Autodesk Inventor part; units mm, degrees
ref_plane "YZ Plane" through (0, 0, 0) normal (1, 0, 0) x (0, 1, 0)
ref_plane "XZ Plane" through (0, 0, 0) normal (0, 1, 0) x (-1, 0, 0)
ref_plane "XY Plane" through (0, 0, 0) normal (0, 0, 1) x (1, 0, 0)
sketch "Sketch1" plane through (0, 0, 0) normal (0, 1, 0) x (-1, 0, 0)
  point P0 (0, 0)
sketch "Sketch2" plane through (0, 0, 0) normal (0, 1, 0) x (-1, 0, 0)
  point P0 (0, 0)
sketch "Sketch3" plane through (0, 0, 0) normal (0, 1, 0) x (-1, 0, 0)
  point P0 (0, 0)
sketch "Sketch4" plane through (0, 0, 0) normal (0, 1, 0) x (-1, 0, 0)
  line L0 (35, 20) -> (-35, 20)
  line L1 (-35, 20) -> (-35, -20)
  line L2 (-35, -20) -> (35, -20)
  line L3 (35, -20) -> (35, 20)
  line L4 (35, 20) -> (-35, -20) construction
  line L5 (-35, 20) -> (35, -20) construction
  point P0 (0, 0)
  dimension "d0" = 70
  dimension "d1" = 40
extrude "Extrusion1" add sketch "Sketch4" along normal blind 2
sketch "Sketch5" plane through (0, 2, 0) normal (0, 1, 0) x (1, 0, 0)
  line L0 (-35, 20) -> (-35, -20)
  line L1 (-35, 0) -> (-25, 0)
  line L2 (-25, 0) -> (-25, 10)
  line L3 (-25, 10) -> (-25, -10)
  circle A0 centre (-25, -10) radius 1.5
  circle A1 centre (-25, 10) radius 1.5
  point P0 (0, 0)
  dimension "d4" = 10
  dimension "d5" = 10
  dimension "d6" = 20
  dimension "d7" = 3
  dimension "d8" = 3
extrude "Extrusion2" cut sketch "Sketch5" against normal blind 3
sketch "Sketch6" plane through (0, 2, 0) normal (0, 1, 0) x (1, 0, 0)
  line L0 (-35, -20) -> (35, -20)
  line L1 (35, 20) -> (-35, 20)
  line L2 (35, -20) -> (-15, -20)
  line L3 (-15, -20) -> (-15, 20)
  line L4 (-15, 20) -> (35, 20)
  line L5 (35, 20) -> (35, -20)
  line L6 (-35, 20) -> (-35, -20)
  line L7 (-15, 20) -> (-35, 20)
  line L8 (-35, 20) -> (-35, 15)
  line L9 (-35, 15) -> (-15, 15)
  line L10 (-15, 15) -> (-15, 20)
  line L11 (-35, -20) -> (-15, -20)
  line L12 (-15, -20) -> (-15, -15)
  line L13 (-15, -15) -> (-35, -15)
  line L14 (-35, -15) -> (-35, -20)
  point P0 (0, 0)
  dimension "d11" = 50
  dimension "d12" = 5
  dimension "d13" = 5
extrude "Extrusion3" add sketch "Sketch6" along normal blind 2 contours L6 L13 L3 L0 | L3 L1 L5 L0 | L6 L1 L3 L9
chamfer "Chamfer1" distance 2 angle 45 3 edges at (-25, 2, 15) (-15, 2, 0) (-25, 2, -15)
sketch "Sketch7" plane through (0, 4, 0) normal (0, 1, 0) x (1, 0, 0)
  line L0 (35, -20) -> (35, 20)
  line L1 (35, -20) -> (28, -20)
  line L2 (28, -20) -> (28, -8)
  line L3 (28, -8) -> (35, -8)
  line L4 (35, -8) -> (35, -20)
  line L5 (35, 20) -> (28, 20)
  line L6 (28, 20) -> (28, 8)
  line L7 (28, 8) -> (35, 8)
  line L8 (35, 8) -> (35, 20)
  point P0 (0, 0)
  dimension "d19" = 7
  dimension "d20" = 12
  dimension "d21" = 12
extrude "Extrusion4" cut sketch "Sketch7" against normal blind 4
sketch "Sketch8" plane through (28, 4, 8) normal (0, 0, 1) x (1, 0, 0)
  line L0 (7, -4) -> (7, 0)
  line L1 (7, 0) -> (3, -4)
  line L2 (0, -4) -> (7, -4)
  line L3 (7, 0) -> (12.6569, 0) construction
  circle A0 centre (5, -2) radius 1.5
  point P0 (-28, -4)
  dimension "d24" = 135
  dimension "d25" = 3
extrude "Extrusion5" add sketch "Sketch8" along normal blind 10 contours A0 L1 | L1 A0
sketch "Sketch9" plane through (35, 4, -8) normal (0, 0, -1) x (-1, 0, 0)
  circle A0 centre (2, -2) radius 1.5
  circle A1 centre (2, -2) radius 1.5
  point P0 (35, -4)
extrude "Extrusion6" add sketch "Sketch9" along normal blind 10
equation "\"d9\" = d7"
properties part number "upper"
The model under review builds one solid part; all positions refer to its coordinate system, in mm. A direction names the side the tool comes from. Round coordinates to 2 decimals unless told otherwise and drop trailing zeros. Loops run counter-clockwise (first coordinate to the right, second up) from the corner with the lowest first, then second, coordinate; pieces in that order, holes last. Notation, with made-up numbers: (-36, 83) -> (-13, 83) arc R32 cw to (-13, 110) -> close; hole circle Ø10 at (45.25, -24.75). An arc over 180 degrees is marked (long way). One line per question, with ' | ' between items. Start each with the question number.
Item 1: Draft analysis for pull direction Z (two halves, no side actions). For faces 1 (the face through (35, 2, 0)), 2 (the face through (-26.5, 1.01, 9.93)), 3 (the face through (31, 2, -8)), 4 (the face through (33, 2, 18)), state which applies: +Z half, -Z half, draft (parallel to the pull), parting line (faces both ways), or undercut.
Item 2: Add section B-B, the plane z = -17. Write out the cut boundary in (x, y), then the cut area to 3 significant figures.
Item 3: Add section A-A, the plane x = -25. Count the separate pieces of the cut face and the enclosed holes in it, then the cut area to 3 significant figures.
Item 4: Wall thickness on line 1 along Z through (x, y) = (-25, 0.65); line 2 along X through (y, z) = (0.75, -10); line 3 along Z through (x, y) = (31, 3.1): over which ranges is each line inside the solid? List them lowest first. Write a range as [from, to].
Item 5: Machinability: for faces 5 (the face through (31.5, 1.93, 12.93)), 6 (the face through (28, 2, 14)), 7 (the face through (-26, 2, 0)), 8 (the face through (34.2, 2.9, -12.9)), 9 (the face through (28, 2, -14)), which of the approach directions +Z, -Z, +X, -X, +Y, -Y give a long, thin tool a straight path to every point of the face, cutting with its end or side? Answer none if there is none.
Item 6: Add section D-D, the plane y = 1.2. Write out the cut boundary in (x, z), then the cut area to 3 significant figures.
Item 7: For pin 1 (2.5 mm diameter, centred on x = -25, z = -10, fed in from +Y); pin 2 (2 mm diameter, centred on x = -22, z = 10.5, fed in from +Y); pin 3 (1.5 mm diameter, centred on y = 3.5, z = -5.5, fed in from -X); pin 4 (1.2 mm diameter, centred on x = 33, y = 2.5, fed in from +Z), all flat-tipped, find the tip position at first contact; note any pin that passes through.
Return value:
1) face 1: draft | face 2: undercut | face 3: -Z half | face 4: +Z half
2) outline: (-35, 0) -> (28, 0) -> (28, 4) -> (-35, 4) -> close; circle Ø3 at (33, 2) | area: 259 mm2
3) separate pieces: 3 | enclosed holes: 0 | area: 92.0 mm2
4) line 1: z = [-20, -11.5], [-8.5, 8.5], [11.5, 20] | line 2: x = [-35, -26.5], [-23.5, 28], [32.17, 33.83] | line 3: z = [-8, 8]
5) face 5: +Z | face 6: +Z, +Y, -Y | face 7: -X, +Y | face 8: -Z | face 9: -Z, +Y, -Y
6) outline: (-35, -20) -> (28, -20) -> (28, -8) -> (31.73, -8) -> (31.73, -18) -> (34.27, -18) -> (34.27, -8) -> (35, -8) -> (35, 8) -> (34.27, 8) -> (34.27, 18) -> (31.73, 18) -> (31.73, 8) -> (28, 8) -> (28, 20) -> (-35, 20) -> close; hole circle Ø3 at (-25, -10); hole circle Ø3 at (-25, 10) | area: 2,670 mm2
7) pin 1: passes through | pin 2: stops at y = 2 | pin 3: stops at x = -16.25 | pin 4: stops at z = 18
